Source: CAD feature listing. Evaluate the final solid. Frame: model axes, mm. A direction names the side the tool comes from. Coordinates: 2 decimals unless noted, no trailing zeros. Write each loop counter-clockwise with the first axis right and the second up, starting at its lowest first coordinate (ties: lowest second). Pieces come first, ordered by that corner, then holes. Notation, with made-up numbers: (4.25, 47.5) - (34.25, 47.5) arc R27 ccw to (34.25, 77.5) - close; hole circle Ø8 at (79.5, 20.5). An arc over 180 degrees is marked (long way). One line per item, written item: value.
from build123d import *

# Parameters (mm, degrees)
SKETCH_1_R              = 28.5
SKETCH_1_R_2            = 6
EXTRUDE_1_DEPTH         = 6
SKETCH_2_R              = 12
SKETCH_2_R_2            = 6
EXTRUDE_2_DEPTH         = 20.5
HOLE_WIZARD_1_4_1_D     = 4.999999906
HOLE_WIZARD_1_4_1_DEPTH = 10
SKETCH_5_R              = 2.5
CUT_EXTRUDE_1_DEPTH     = 30
CUT_EXTRUDE_START       = -100
CUT_EXTRUDE_2_DEPTH     = 100


with BuildPart() as part:
    # ｽｹｯﾁ1 → ﾎﾞｽ - 押し出し1 (new body)
    with BuildSketch(Plane.XY):
        Circle(SKETCH_1_R)
        Circle(SKETCH_1_R_2, mode=Mode.SUBTRACT)
    extrude(amount=EXTRUDE_1_DEPTH)

    # ｽｹｯﾁ2 → ﾎﾞｽ - 押し出し2 (add)
    with BuildSketch(Plane.XY.offset(6)):
        Circle(SKETCH_2_R)
        Circle(SKETCH_2_R_2, mode=Mode.SUBTRACT)
    extrude(amount=EXTRUDE_2_DEPTH)

    # 1/4 すきま穴1
    with Locations(Plane(origin=(11.999037225, 0.152005526, 19.728327371), x_dir=(-0.012667127201, 0.999919768726, 0), z_dir=(0.999919768726, 0.012667127201, 0))):
        with Locations((0, 0)):
            Hole(HOLE_WIZARD_1_4_1_D / 2, depth=HOLE_WIZARD_1_4_1_DEPTH)

    # ｽｹｯﾁ5 → ｶｯﾄ - 押し出し1 (cut)
    with BuildSketch(Plane.XY.offset(6)):
        with BuildLine():
            ThreePointArc((-17.851596989, 11.75), (-17.936782423, 12.397047613), (-18.186533479, 13))
            Line((-18.186533479, 13), (-20.351596989, 11.75))
            Line((-20.351596989, 11.75), (-20.351596989, 9.25))
            ThreePointArc((-20.351596989, 9.25), (-18.583830036, 9.982233047), (-17.851596989, 11.75))
        make_face()
        with BuildLine():
            Line((-20.351596989, 11.75), (-18.186533479, 13))
            ThreePointArc((-18.186533479, 13), (-22.516660498, 13), (-20.351596989, 9.25))
            Line((-20.351596989, 9.25), (-20.351596989, 11.75))
        make_face()
        with BuildLine():
            ThreePointArc((22.851596989, 11.75), (20.998644602, 14.164814566), (18.186533479, 13))
            Line((18.186533479, 13), (20.351596989, 11.75))
            Line((20.351596989, 11.75), (20.351596989, 9.25))
            ThreePointArc((20.351596989, 9.25), (22.119363942, 9.982233047), (22.851596989, 11.75))
        make_face()
        with BuildLine():
            Line((20.351596989, 11.75), (18.186533479, 13))
            ThreePointArc((18.186533479, 13), (18.186533479, 10.5), (20.351596989, 9.25))
            Line((20.351596989, 9.25), (20.351596989, 11.75))
        make_face()
        with Locations((0, 23.5)):
            Circle(SKETCH_5_R)
        with Locations((-20.351596989, -11.75)):
            Circle(SKETCH_5_R)
        with Locations((0, -23.5)):
            Circle(SKETCH_5_R)
        with Locations((20.351596989, -11.75)):
            Circle(SKETCH_5_R)
    extrude(amount=-CUT_EXTRUDE_1_DEPTH, mode=Mode.SUBTRACT)

    # ｽｹｯﾁ6 → ｶｯﾄ - 押し出し2 (cut)
    with BuildSketch(Plane.XY.offset(26.5).offset(CUT_EXTRUDE_START)):
        with BuildLine():
            Line((-2, 7.4), (-2, 5.656854249))
            ThreePointArc((-2, 5.656854249), (0, 6), (2, 5.656854249))
            Line((2, 5.656854249), (2, 7.4))
            Line((2, 7.4), (-2, 7.4))
        make_face()
    extrude(amount=CUT_EXTRUDE_2_DEPTH, mode=Mode.SUBTRACT)


solid = part.part
1) Material intervals for line 1 (Y direction, x = 0, z = 2.6); line 2 (Y direction, x = 0, z = 18.5); line 3 (X direction, y = 11.75, z = 2.6), sorted ascending.
Values found:
line 1: -28.5 to -26, -21 to -6, 7.4 to 21, 26 to 28.5
line 2: -12 to -6, 7.4 to 12
line 3: -25.97 to -22.85, -17.85 to 17.85, 22.85 to 25.97
2) Draft query along Y for faces 1 (the cylindrical face through (26.327, -10.916, 2.958)), 2 (the flat face through (-7, 0, 0)), 3 (the flat face through (-2, 7, 13)). Return one class per face: released by +Y, released by -Y, zero draft, split by the parting line, or undercut.
Values found:
face 1: split by the parting line
face 2: zero draft
face 3: undercut
3) Section query C-C on z = 10.75. Output: boundary loops of the cut face in (x, y).
Values found:
outline: circle Ø24 at (0, 0); hole (-2, 5.66) arc R6 ccw (long way) to (2, 5.66) - (2, 7.4) - (-2, 7.4) - close
4) Section query A-A on x = 0. Output: boundary loops of the cut face in (y, z), then the cut area to 3 significant figures.
Values found:
outline: (-28.5, 0) - (-26, 0) - (-26, 6) - (-28.5, 6) - close; (-21, 0) - (-6, 0) - (-6, 26.5) - (-12, 26.5) - (-12, 6) - (-21, 6) - close; (7.4, 0) - (21, 0) - (21, 6) - (12, 6) - (12, 26.5) - (7.4, 26.5) - close; (26, 0) - (28.5, 0) - (28.5, 6) - (26, 6) - close
area: 419 mm2
5) Contact query for flat-ended pins moving along their axis: P1, Ø3, axis at y = -1.5, z = 14, coming from the +X side; P2, Ø1.9, axis at y = 7, z = 9, coming from the +X side; P3, Ø8, axis at y = 4.5, z = 5, coming from the -X side. Output: stop coordinate, or through.
Values found:
P1: x = 12
P2: x = 10.36
P3: x = -28.5
6) Section query B-B on y = -24.5. Output: boundary loops of the cut face in (x, z), then the cut area to 3 significant figures.
Values found:
outline: (-14.56, 0) - (-2.29, 0) - (-2.29, 6) - (-14.56, 6) - close; (2.29, 0) - (14.56, 0) - (14.56, 6) - (2.29, 6) - close
area: 147 mm2
7) Reachability of faces 4 (the flat face through (0, 7.4, 13)), 5 (the cylindrical face through (-11.99, 0.53, 16.11)), 6 (the cylindrical face through (8.651, 2.607, 19.838)) from +Z, -Z, +X, -X, +Y, -Y: full face, straight path, thin tool, end or side. Return the list, or none.
Values found:
face 4: +Z, -Z
face 5: +Z
face 6: none
8) Section query D-D on x = -19. Output: boundary loops of the cut face in (y, z).
Values found:
outline: (-21.24, 0) - (-13.85, 0) - (-13.85, 6) - (-21.24, 6) - close; (-9.65, 0) - (9.65, 0) - (9.65, 6) - (-9.65, 6) - close; (13.85, 0) - (21.24, 0) - (21.24, 6) - (13.85, 6) - close
